```python
from build123d import *

# Parameters (mm, degrees)
SKETCH1_W           = 53
SKETCH1_H           = 7
BOSS_EXTRUDE1_DEPTH = 2
SKETCH2_R           = 1.5
CUT_EXTRUDE1_DEPTH  = 2
SKETCH3_W           = 53
SKETCH3_H           = 7
BOSS_EXTRUDE2_DEPTH = 10
SKETCH4_R           = 2
CUT_EXTRUDE2_DEPTH  = 3.5


with BuildPart() as part:
    # Sketch1 → Boss-Extrude1 (new body)
    with BuildSketch(Plane(origin=(0, 0, 0), x_dir=(1, 0, 0), z_dir=(0, 1, 0))):
        with BuildLine():
            Line((3.5, 15), (0.251527995, 7.574921132))
            ThreePointArc((0.251527995, 7.574921132), (0.144442027, 7.29213232), (0.066367549, 7))
            Line((0.066367549, 7), (59.933632451, 7))
            ThreePointArc((59.933632451, 7), (59.855557973, 7.29213232), (59.748472005, 7.574921132))
            Line((59.748472005, 7.574921132), (56.5, 15))
            Line((56.5, 15), (3.5, 15))
        make_face()
        with Locations((30, 18.5)):
            Rectangle(SKETCH1_W, SKETCH1_H)
        with BuildLine():
            Line((59.933632451, 7), (0.066367549, 7))
            ThreePointArc((0.066367549, 7), (0.016638024, 6.687982178), (0, 6.37246463))
            Line((0, 6.37246463), (0, 3))
            ThreePointArc((0, 3), (0.878679656, 0.878679656), (3, 0))
            Line((3, 0), (57, 0))
            ThreePointArc((57, 0), (59.121320344, 0.878679656), (60, 3))
            Line((60, 3), (60, 6.37246463))
            ThreePointArc((60, 6.37246463), (59.983361976, 6.687982178), (59.933632451, 7))
        make_face()
    extrude(amount=BOSS_EXTRUDE1_DEPTH)

    # Sketch2 → Cut-Extrude1 (cut)
    with BuildSketch(Plane(origin=(0, 2, 0), x_dir=(1, 0, 0), z_dir=(0, 1, 0))):
        with Locations(Location((3.5, 3.5, 0), (0, 0, 270))):
            Circle(SKETCH2_R)
        with Locations(Location((56.5, 3.5, 0), (0, 0, 270))):
            Circle(SKETCH2_R)
    extrude(amount=-CUT_EXTRUDE1_DEPTH, mode=Mode.SUBTRACT)

    # Sketch3 → Boss-Extrude2 (add)
    with BuildSketch(Plane(origin=(0, 2, 0), x_dir=(1, 0, 0), z_dir=(0, 1, 0))):
        with Locations((30, 18.5)):
            Rectangle(SKETCH3_W, SKETCH3_H)
    extrude(amount=BOSS_EXTRUDE2_DEPTH)

    # Sketch4 → Cut-Extrude2 (cut)
    with BuildSketch(Plane(origin=(0, 12, 0), x_dir=(1, 0, 0), z_dir=(0, 1, 0))):
        with Locations(Location((7, 18.5, 0), (0, 0, 270))):
            Circle(SKETCH4_R)
        with Locations(Location((53, 18.5, 0), (0, 0, 270))):
            Circle(SKETCH4_R)
    extrude(amount=-CUT_EXTRUDE2_DEPTH, mode=Mode.SUBTRACT)


solid = part.part
```
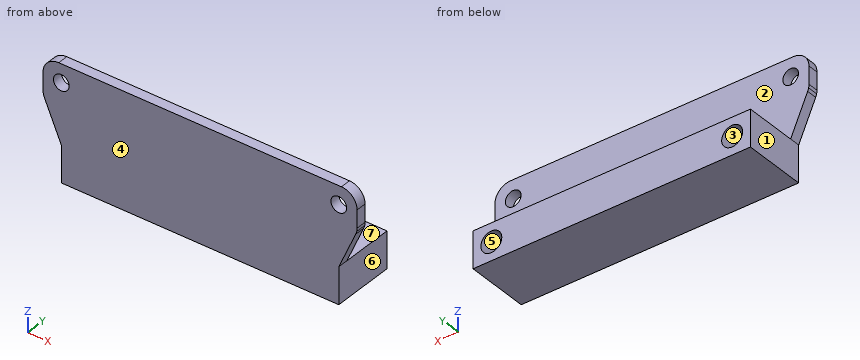
Work out the finished part from the listing and answer in its coordinate system (mm). Face numbers are marked on the shaded views. A direction names the side the tool comes from. Give positions to 0.01 mm unless a question says otherwise; leave off trailing zeros. Write each loop counter-clockwise with the first axis right and the second up, starting at its lowest first coordinate (ties: lowest second). Pieces come first, ordered by that corner, then holes.
(1) Straight lines are drawn through the part: line 1 (X direction, y = 9.35, z = -18.5); line 2 (X direction, y = 1.65, z = -3.5); line 3 (Y direction, x = 29, z = -14.75). For each, find the intervals that lie inside material, in ascending order.
Final values:
line 1: x = 3.5 to 5, 9 to 51, 55 to 56.5
line 2: x = 0 to 2, 5 to 55, 58 to 60
line 3: y = 0 to 2
(2) The part is cut by section A-A on z = -18.5. Write down the section's boundary in (x, y).
Final values:
outline: (3.5, 0) - (56.5, 0) - (56.5, 12) - (55, 12) - (55, 8.5) - (51, 8.5) - (51, 12) - (9, 12) - (9, 8.5) - (5, 8.5) - (5, 12) - (3.5, 12) - close
(3) Flat-ended cylindrical pins translate along their axes: pin 1 Ø6 at (x, z) = (52.5, -4.5) entering from +Y; pin 2 Ø5.5 at (y, z) = (5, -17.5) entering from +X; pin 3 Ø5 at (x, y) = (44, 9) entering from +Z. Find the tip coordinate at first contact, or state that the pin passes through.
Final values:
pin 1: stops at y = 2
pin 2: stops at x = 56.5
pin 3: stops at z = -15
(4) The part is cut by section B-B on y = 9.5. Write down the section's boundary in (x, z).
Final values:
outline: (3.5, -22) - (56.5, -22) - (56.5, -15) - (3.5, -15) - close; hole circle Ø4 at (7, -18.5); hole circle Ø4 at (53, -18.5)
(5) The part is cut by section C-C on x = 7. Write down the section's boundary in (y, z), plus the area to 3 significant figures.
Final values:
outline: (0, -22) - (12, -22) - (12, -20.5) - (8.5, -20.5) - (8.5, -16.5) - (12, -16.5) - (12, -15) - (2, -15) - (2, 0) - (0, 0) - close
area: 100 mm2
(6) The part is cut by section D-D on y = 3.5. Write down the section's boundary in (x, z), plus the area to 3 significant figures.
Final values:
outline: (3.5, -22) - (56.5, -22) - (56.5, -15) - (3.5, -15) - close
area: 371 mm2
(7) Which of the six approach directions +Z, -Z, +X, -X, +Y, -Y give full straight-line access (tool end or side, diameter ignored) to the marked faces 1, 2, 3 and 4?
Final values:
face 1: -Z, -X, +Y, -Y
face 2: +Z, +X, -X, +Y
face 3: +Y
face 4: +Z, -Z, +X, -X, -Y
(8) The mould has two halves that part along Z. Classify the marked faces 5, 6 and 7: pulls with the +Z half, pulls with the -Z half, needs draft (parallel to the pull), parting line crosses it, or undercut.
Final values:
face 5: undercut
face 6: needs draft
face 7: pulls with the +Z half
